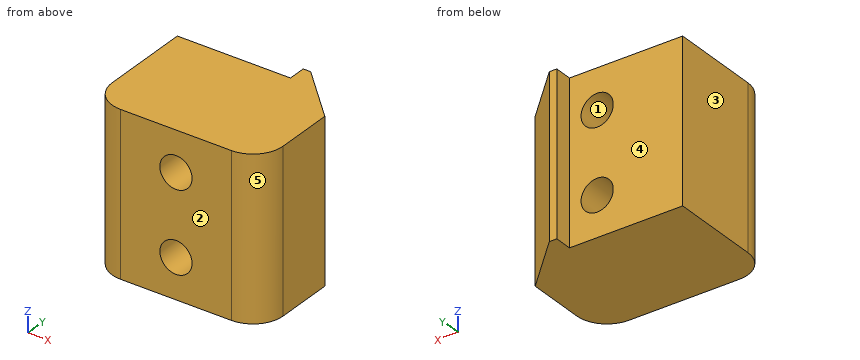
from build123d import *

# Parameters (mm, degrees)
CYLINDER898_R          = 1.6
CYLINDER898_DEPTH      = 20
CYLINDER898_ROLL_ANGLE = 90
CYLINDER897_R          = 1.6
CYLINDER897_DEPTH      = 20
CYLINDER897_ROLL_ANGLE = 90
BOX552_W               = 17
BOX552_H               = 12
BOX552_DEPTH           = 16
BOX553_W               = 5.75
BOX553_H               = 1.75
BOX553_DEPTH           = 16
CHAMFER001_SIZE        = 5
FILLET013_R            = 3


with BuildPart() as cylinder1021:
    # Cylinder898 → Cylinder898 (new body)
    with BuildSketch(Plane.XY):
        Circle(CYLINDER898_R)
    extrude(amount=CYLINDER898_DEPTH)


with BuildPart() as cylinder1021_1:
    # Cylinder898 roll: moved
    add(cylinder1021.part.rotate(Axis((0, 0, 0), (1, 0, 0)), CYLINDER898_ROLL_ANGLE))


with BuildPart() as cylinder1021_2:
    # Cylinder898 placement: moved
    add(cylinder1021_1.part.moved(Location((19.5, 30, 0.5))))


with BuildPart() as fusion056:
    # Cylinder897 → Cylinder897 (new body)
    with BuildSketch(Plane.XY):
        Circle(CYLINDER897_R)
    extrude(amount=CYLINDER897_DEPTH)


with BuildPart() as fusion056_1:
    # Cylinder897 roll: moved
    add(fusion056.part.rotate(Axis((0, 0, 0), (1, 0, 0)), CYLINDER897_ROLL_ANGLE))


with BuildPart() as fusion056_2:
    # Cylinder897 placement: moved
    add(fusion056_1.part.moved(Location((19.5, 30, -7.5))))

    # Fusion056: union Cylinder1021
    add(cylinder1021_2.part)


with BuildPart() as fusion056_3:
    # Fusion056 placement: moved
    add(fusion056_2.part.moved(Location((0, -40, 0))))


with BuildPart() as cube743:
    # Box552 → Box552 (new body)
    with BuildSketch(Plane(origin=(11, -30, -11.5), x_dir=(1, 0, 0), z_dir=(0, 0, 1))):
        with Locations((8.5, 6)):
            Rectangle(BOX552_W, BOX552_H)
    extrude(amount=BOX552_DEPTH)


with BuildPart() as diff_box_mount_left:
    # Box553 → Box553 (new body)
    with BuildSketch(Plane(origin=(22.25, -18, -11.5), x_dir=(1, 0, 0), z_dir=(0, 0, 1))):
        with Locations((2.875, 0.875)):
            Rectangle(BOX553_W, BOX553_H)
    extrude(amount=BOX553_DEPTH)

    # Fusion055: union Cube743
    add(cube743.part)

    # Chamfer001
    chamfer001_edges = [diff_box_mount_left.edges().sort_by_distance(p)[0] for p in [
        (28, -16.25, -3.5),
    ]]
    chamfer(chamfer001_edges, length=CHAMFER001_SIZE)

    # Fillet013
    fillet013_edges = [diff_box_mount_left.edges().sort_by_distance(p)[0] for p in [
        (28, -30, -3.5),
        (11, -30, -3.5),
    ]]
    fillet(fillet013_edges, radius=FILLET013_R)

    # Cut014020: cut Fusion056
    add(fusion056_3.part, mode=Mode.SUBTRACT)


with BuildPart() as diff_box_mount_left_1:
    # Cut014020 placement: moved
    add(diff_box_mount_left.part.moved(Location((0, 0, -1))))


solid = diff_box_mount_left_1.part
Build history of the part. All positions in model axes, mm. Face numbers are marked on the shaded views. A direction names the side the tool comes from. Round coordinates to 2 decimals unless told otherwise and drop trailing zeros. Write each loop counter-clockwise with the first axis right and the second up, starting at its lowest first coordinate (ties: lowest second). Pieces come first, ordered by that corner, then holes. Notation, with made-up numbers: (-36.5, -24) - (-3.5, -24) arc R21 ccw to (-3.5, -4) - close; hole circle Ø3 at (48, 14.5). An arc over 180 degrees is marked (long way). Use CSV: the item, a comma, the result in double quotes.
(1) Band-saw the part on A-A (z = -8.5). Write the cut outline in (x, y).
Response:
outline,"(11, -27) arc R3 ccw to (14, -30) - (17.9, -30) - (17.9, -18) - (11, -18) - close; (21.1, -30) - (25, -30) arc R3 ccw to (28, -27) - (28, -21.25) - (23, -16.25) - (22.25, -16.25) - (22.25, -18) - (21.1, -18) - close"
(2) Band-saw the part on D-D (y = -21.5). Write the cut outline in (x, z), plus the area to 3 significant figures.
Response:
outline,"(11, -12.5) - (28, -12.5) - (28, 3.5) - (11, 3.5) - close; hole circle Ø3.2 at (19.5, -8.5); hole circle Ø3.2 at (19.5, -0.5)"
area,"256 mm²"
(3) Wall check: line 1 (Z direction, x = 19.5, y = -25.5); line 2 (X direction, y = -26, z = -8.5); line 3 (Z direction, x = 18.75, y = -22.75). Give the ranges that are in metal, low to high.
Response:
line 1,"-12.5 to -10.1, -6.9 to -2.1, 1.1 to 3.5"
line 2,"11 to 17.9, 21.1 to 28"
line 3,"-12.5 to -9.91, -7.09 to -1.91, 0.91 to 3.5"
(4) Mould opens along X. For the marked faces 1, 2 and 3 say: pulls with the +X half, pulls with the -X half, needs draft (parallel to the pull), parting line crosses it, or undercut.
Response:
face 1,"undercut"
face 2,"needs draft"
face 3,"pulls with the -X half"
(5) Band-saw the part on B-B (x = 19.5). Write the cut outline in (y, z).
Response:
outline,"(-30, -12.5) - (-18, -12.5) - (-18, -10.1) - (-30, -10.1) - close; (-30, -6.9) - (-18, -6.9) - (-18, -2.1) - (-30, -2.1) - close; (-30, 1.1) - (-18, 1.1) - (-18, 3.5) - (-30, 3.5) - close"
(6) 3-axis set-ups, long thin cutter, end or side, ignore diameter. For the marked faces 4 and 5: which of +Z, -Z, +X, -X, +Y, -Y reach the whole face in a straight line?
Response:
face 4,"+Z, -Z, -X, +Y"
face 5,"+Z, -Z, +X, -Y"
(7) Band-saw the part on C-C (z = 1.75). Write the cut outline in (x, y), plus the area to 3 significant figures.
Response:
outline,"(11, -27) arc R3 ccw to (14, -30) - (25, -30) arc R3 ccw to (28, -27) - (28, -21.25) - (23, -16.25) - (22.25, -16.25) - (22.25, -18) - (11, -18) - close"
area,"198 mm²"
(8) Pin check, flat tips, straight feed: P1, Ø3, axis at x = 21.5, z = 0, coming from the +Y side; P2, Ø9, axis at x = 17, z = -2.5, coming from the +Y side; P3, Ø1.9, axis at y = -17, z = -4.5, coming from the -X side; P4, Ø1.5, axis at x = 26, z = -4, coming from the +Y side. Stop position of each tip, or through.
Response:
P1,"y = -16.25"
P2,"y = -18"
P3,"x = 22.25"
P4,"y = -18.5"
